from build123d import *

# Parameters (mm, degrees)
EXTRUDE_1_DEPTH     = 7
SKETCH_2_R          = 20
CUT_EXTRUDE_1_DEPTH = 7
SKETCH_3_R          = 1.6
CUT_EXTRUDE_2_DEPTH = 7
FILLET_1_R          = 5
SKETCH_4_R          = 1.25
CUT_EXTRUDE_3_DEPTH = 10


with BuildPart() as part:
    # 草图1 → 凸台-拉伸1 (new body)
    with BuildSketch(Plane.XY):
        with BuildLine():
            ThreePointArc((-24.633500506, 4.265050152), (0, 25), (24.633500506, 4.265050152))
            Line((24.633500506, 4.265050152), (60, -200))
            Line((60, -200), (-60, -200))
            Line((-60, -200), (-24.633500506, 4.265050152))
        make_face()
    extrude(amount=EXTRUDE_1_DEPTH)

    # 草图2 → 切除-拉伸1 (cut)
    with BuildSketch(Plane.XY.offset(7)):
        Circle(SKETCH_2_R)
    extrude(amount=-CUT_EXTRUDE_1_DEPTH, mode=Mode.SUBTRACT)

    # 草图3 → 切除-拉伸2 (cut)
    with BuildSketch(Plane.XY.offset(7)):
        with Locations((-15.001714002, -194)):
            Circle(SKETCH_3_R)
        with Locations((14.998285998, -194)):
            Circle(SKETCH_3_R)
    extrude(amount=-CUT_EXTRUDE_2_DEPTH, mode=Mode.SUBTRACT)

    # 圆角1
    fillet_1_edges = [part.edges().sort_by_distance(p)[0] for p in [
        (60, -200, 3.5),
        (-60, -200, 3.5),
    ]]
    fillet(fillet_1_edges, radius=FILLET_1_R)

    # 草图4 → 切除-拉伸3 (cut)
    with BuildSketch(Plane.XY.offset(7)):
        with Locations((-50.001714002, -197)):
            Circle(SKETCH_4_R)
        with Locations((-30.001714002, -197)):
            Circle(SKETCH_4_R)
        with Locations((30.001714002, -197)):
            Circle(SKETCH_4_R)
        with Locations((50.001714002, -197)):
            Circle(SKETCH_4_R)
    extrude(amount=-CUT_EXTRUDE_3_DEPTH, mode=Mode.SUBTRACT)


solid = part.part
Can you work these out from the model? Positions are in its coordinate system, mm. Round coordinates to 2 decimals unless told otherwise and drop trailing zeros. Write each loop counter-clockwise with the first axis right and the second up, starting at its lowest first coordinate (ties: lowest second). Pieces come first, ordered by that corner, then holes. Notation, with made-up numbers: (62.5, 51) -> (121.5, 51) arc R16 ccw to (121.5, 79) -> close; hole circle Ø9 at (-25.5, -29). An arc over 180 degrees is marked (long way). Use one line per item in the form item = value. Start each with the question number.
Q1. We'd pull the mould along Z, two halves only. Please class faces 1 (the face through (1, -111, 7)), 2 (the face through (41.57, -93.55, 3.45)), 3 (the face through (1, -111, 0)): +Z half, -Z half, draft (parallel to the pull), parting line (faces both ways), or undercut.
Q2. Imagine slicing it at C-C (y = 0). Please give me the cut outline in (x, z).
Q3. If I drill on probe 1 along X at (y, z) = (-194, 5.5); probe 2 along X at (y, z) = (-197, 5); probe 3 along Y at (x, z) = (14, 2.5), over which ranges is the centre line in solid material (lowest first)? Write a range as [from, to].
Q4. Imagine slicing it at D-D (y = -91). Please give me the cut outline in (x, z), then the cut area to 3 significant figures.
Q5. I'm going to push a flat-ended pin straight in: P1, Ø4, axis at x = -15, y = -194, coming from the -Z side. Where does the tip first touch, or does it pass through?
Q6. Imagine slicing it at A-A (x = 0). Please give me the cut outline in (y, z), then the cut area to 4 significant figures.
Q7. Imagine slicing it at B-B (z = 5.75). Please give me the cut outline in (x, y).
Worked out:
q1.face_1 = +Z half
q1.face_2 = draft
q1.face_3 = -Z half
q2.outline = (-25.37, 0) -> (-20, 0) -> (-20, 7) -> (-25.37, 7) -> close; (20, 0) -> (25.37, 0) -> (25.37, 7) -> (20, 7) -> close
q3.probe_1 = [-58.96, -16.6], [-13.4, 13.4], [16.6, 58.96]
q3.probe_2 = [-58.64, -51.25], [-48.75, -31.25], [-28.75, 28.75], [31.25, 48.75], [51.25, 58.64]
q3.probe_3 = [-200, -195.25], [-192.75, -14.28], [14.28, 20.71]
q4.outline = (-41.13, 0) -> (41.13, 0) -> (41.13, 7) -> (-41.13, 7) -> close
q4.area = 576 mm^2
q5.P1 = 0
q6.outline = (-200, 0) -> (-20, 0) -> (-20, 7) -> (-200, 7) -> close; (20, 0) -> (25, 0) -> (25, 7) -> (20, 7) -> close
q6.area = 1,295 mm^2
q7.outline = (-58.99, -194.15) arc R5 ccw to (-54.06, -200) -> (54.06, -200) arc R5 ccw to (58.99, -194.15) -> (24.63, 4.27) arc R25 ccw to (-24.63, 4.27) -> close; hole circle Ø2.5 at (-50, -197); hole circle Ø2.5 at (-30, -197); hole circle Ø40 at (0, 0); hole circle Ø3.2 at (-15, -194); hole circle Ø3.2 at (15, -194); hole circle Ø2.5 at (30, -197); hole circle Ø2.5 at (50, -197)
